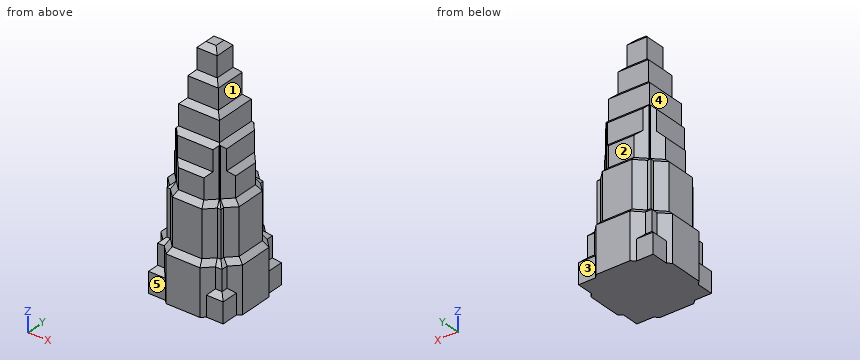
from build123d import *

# Parameters (mm, degrees)
F1_DEPTH     = 25.4
F2_SIZE      = 5.08
F3_DEPTH     = 25.4
F4_SIZE      = 5.08
F5_DEPTH     = 25.4
F6_DEPTH     = 25.4
F7_SIZE      = 5.08
F8_DEPTH     = 25.4
F9_SIZE      = 5.08
F10_DEPTH    = 25.4
F11_T1_DEPTH = 61.5024806542
F11_T3_DEPTH = 61.5024806542
F12_DEPTH    = 25.4
F13_SIZE     = 5.08
F14_DEPTH    = 25.4
F15_SIZE     = 5.08
F16_DEPTH    = 25.4
F17_SIZE     = 5.08


# Not quite as in the source:
# - a fillet or chamfer that OpenCascade refuses, or shapes differently, is made with other operations: its cross-section is extruded or revolved along the edge and cut away or added


with BuildPart() as f1:
    # F0 (on Top) → F1 (new body)
    with BuildSketch(Plane.XY):
        Polygon((37.0489656925, 20.3627443159), (37.0489656925, 37.0489656925), (20.3627443159, 37.0489656925), align=None)
        Polygon((40.5962094665, 16.8155005419), (37.0489656925, 20.3627443159), (37.0489656925, -20.3627443159), (40.5962094665, -16.8155005419), align=None)
        Polygon((37.0489656925, -20.3627443159), (37.0489656925, 20.3627443159), (20.3627443159, 37.0489656925), (-20.3627443159, 37.0489656925), (-37.0489656925, 20.3627443159), (-37.0489656925, -20.3627443159), (-20.3627443159, -37.0489656925), (20.3627443159, -37.0489656925), align=None)
        Polygon((-20.3627443159, 37.0489656925), (20.3627443159, 37.0489656925), (16.8155005419, 40.5962094665), (-16.8155005419, 40.5962094665), align=None)
        Polygon((37.0489656925, -37.0489656925), (37.0489656925, -20.3627443159), (20.3627443159, -37.0489656925), align=None)
        Polygon((-37.0489656925, 20.3627443159), (-20.3627443159, 37.0489656925), (-37.0489656925, 37.0489656925), align=None)
        Polygon((16.8155005419, -40.5962094665), (20.3627443159, -37.0489656925), (-20.3627443159, -37.0489656925), (-16.8155005419, -40.5962094665), align=None)
        Polygon((-37.0489656925, -20.3627443159), (-37.0489656925, 20.3627443159), (-40.5962094665, 16.8155005419), (-40.5962094665, -16.8155005419), align=None)
        Polygon((-37.0489656925, -37.0489656925), (-20.3627443159, -37.0489656925), (-37.0489656925, -20.3627443159), align=None)
    extrude(amount=F1_DEPTH)

    # F2
    f2_edges = [f1.edges().sort_by_distance(p)[0] for p in [
        (-28.705855, 37.048966, 25.4),
        (-37.048966, 28.705855, 25.4),
        (28.705855, 37.048966, 25.4),
        (37.048966, 28.705855, 25.4),
        (37.048966, -28.705855, 25.4),
        (28.705855, -37.048966, 25.4),
        (-28.705855, -37.048966, 25.4),
        (-37.048966, -28.705855, 25.4),
    ]]
    chamfer(f2_edges, length=F2_SIZE)

    # F3 (add): a face of the model
    f3_faces = [f1.faces().sort_by_distance(p)[0] for p in [
        (0, 0, 25.4),
    ]]
    extrude(f3_faces, amount=F3_DEPTH)

    # F4
    f4_edges = [f1.edges().sort_by_distance(p)[0] for p in [
        (-21.129122, 36.282588, 50.8),
        (-28.705855, 31.968966, 50.8),
        (-31.968966, 28.705855, 50.8),
        (-36.282588, 21.129122, 50.8),
        (-40.596209, 0, 50.8),
        (-36.282588, -21.129122, 50.8),
        (-31.968966, -28.705855, 50.8),
        (-28.705855, -31.968966, 50.8),
        (-21.129122, -36.282588, 50.8),
        (0, -40.596209, 50.8),
        (21.129122, -36.282588, 50.8),
        (28.705855, -31.968966, 50.8),
        (31.968966, -28.705855, 50.8),
        (36.282588, -21.129122, 50.8),
        (40.596209, 0, 50.8),
        (36.282588, 21.129122, 50.8),
        (31.968966, 28.705855, 50.8),
        (28.705855, 31.968966, 50.8),
        (21.129122, 36.282588, 50.8),
        (0, 40.596209, 50.8),
    ]]
    chamfer(f4_edges, length=F4_SIZE)

    # F5 (add): a face of the model
    f5_faces = [f1.faces().sort_by_distance(p)[0] for p in [
        (0, 0, 50.8),
    ]]
    extrude(f5_faces, amount=F5_DEPTH)

    # F6 (add): a face of the model
    f6_faces = [f1.faces().sort_by_distance(p)[0] for p in [
        (0, 0, 76.2),
    ]]
    extrude(f6_faces, amount=F6_DEPTH)

    # F7
    f7_edges = [f1.edges().sort_by_distance(p)[0] for p in [
        (-19.024918, 31.202588, 101.6),
        (-25.113753, 26.888966, 101.6),
        (0, 35.516209, 101.6),
        (-26.888966, 25.113753, 101.6),
        (19.024918, 31.202588, 101.6),
        (-31.202588, 19.024918, 101.6),
        (25.113753, 26.888966, 101.6),
        (-35.516209, 0, 101.6),
        (26.888966, 25.113753, 101.6),
        (-31.202588, -19.024918, 101.6),
        (31.202588, 19.024918, 101.6),
        (-26.888966, -25.113753, 101.6),
        (35.516209, 0, 101.6),
        (-25.113753, -26.888966, 101.6),
        (31.202588, -19.024918, 101.6),
        (-19.024918, -31.202588, 101.6),
        (26.888966, -25.113753, 101.6),
        (0, -35.516209, 101.6),
        (25.113753, -26.888966, 101.6),
        (19.024918, -31.202588, 101.6),
    ]]
    chamfer(f7_edges, length=F7_SIZE)

    # F8 (add): a face of the model
    f8_faces = [f1.faces().sort_by_distance(p)[0] for p in [
        (0, 0, 101.6),
    ]]
    extrude(f8_faces, amount=F8_DEPTH)

    # F9
    f9_edges = [f1.edges().sort_by_distance(p)[0] for p in [
        (0, 30.436209, 127),
        (-30.436209, 0, 127),
        (30.436209, 0, 127),
        (0, -30.436209, 127),
    ]]
    chamfer(f9_edges, length=F9_SIZE)

    # F10 (add): a face of the model
    f10_faces = [f1.faces().sort_by_distance(p)[0] for p in [
        (0, 0, 127),
    ]]
    extrude(f10_faces, amount=F10_DEPTH)

    # F11: chamfer of 5.08 on 4 edges, made by hand

    # F11_s2 → F11_t1 (cut)
    with BuildSketch(Plane.XZ.offset(-30.7512403271)):
        Polygon((-25.3562094665, 147.32), (-20.2762094665, 152.4), (-25.3562094665, 152.4), align=None)
        Polygon((25.3562094665, 147.32), (20.2762094665, 152.4), (25.3562094665, 152.4), align=None)
    extrude(amount=F11_T1_DEPTH, mode=Mode.SUBTRACT)

    # F11_s4 → F11_t3 (cut)
    with BuildSketch(Plane.YZ.offset(-30.7512403271)):
        Polygon((-25.3562094665, 147.32), (-20.2762094665, 152.4), (-25.3562094665, 152.4), align=None)
        Polygon((20.2762094665, 152.4), (25.3562094665, 147.32), (25.3562094665, 152.4), align=None)
    extrude(amount=F11_T3_DEPTH, mode=Mode.SUBTRACT)

    # F12 (add): a face of the model
    f12_faces = [f1.faces().sort_by_distance(p)[0] for p in [
        (0, 0, 152.4),
    ]]
    extrude(f12_faces, amount=F12_DEPTH)

    # F13
    f13_edges = [f1.edges().sort_by_distance(p)[0] for p in [
        (0, 20.276209, 177.8),
        (20.276209, 0, 177.8),
        (0, -20.276209, 177.8),
        (-20.276209, 0, 177.8),
    ]]
    chamfer(f13_edges, length=F13_SIZE)

    # F14 (add): a face of the model
    f14_faces = [f1.faces().sort_by_distance(p)[0] for p in [
        (0, 0, 177.8),
    ]]
    extrude(f14_faces, amount=F14_DEPTH)

    # F15
    f15_edges = [f1.edges().sort_by_distance(p)[0] for p in [
        (0, 15.196209, 203.2),
        (-15.196209, 0, 203.2),
        (15.196209, 0, 203.2),
        (0, -15.196209, 203.2),
    ]]
    chamfer(f15_edges, length=F15_SIZE)

    # F16 (add): a face of the model
    f16_faces = [f1.faces().sort_by_distance(p)[0] for p in [
        (0, 0, 203.2),
    ]]
    extrude(f16_faces, amount=F16_DEPTH)

    # F17
    f17_edges = [f1.edges().sort_by_distance(p)[0] for p in [
        (0, 10.116209, 228.6),
        (-10.116209, 0, 228.6),
        (10.116209, 0, 228.6),
        (0, -10.116209, 228.6),
    ]]
    chamfer(f17_edges, length=F17_SIZE)


solid = f1.part
CAD build for the part. Positions are in the model's coordinates, mm. Face numbers are marked on the shaded views. A direction names the side the tool comes from. Give positions to 0.01 mm unless a question says otherwise; leave off trailing zeros. Order: outer loops, then holes, each group sorted by start corner. A loop starts at its lowest first (then second) coordinate and runs counter-clockwise, first axis right, second up. Notation, with made-up numbers: (37.5, -3.75) - (63.5, -3.75) arc R21 ccw to (63.5, 4.25) - close; hole circle Ø6 at (83.5, 78.25). An arc over 180 degrees is marked (long way). Answer in a Markdown table with one row per item.
1. Saw through at B-B, the plane z = 74. Give the cut face in (x, y), plus the area to 3 significant figures.
Data:
| item | result |
|---|---|
| outline | (-35.52, -14.71) - (-26.89, -23.34) - (-26.89, -26.89) - (-23.34, -26.89) - (-14.71, -35.52) - (14.71, -35.52) - (23.34, -26.89) - (26.89, -26.89) - (26.89, -23.34) - (35.52, -14.71) - (35.52, 14.71) - (26.89, 23.34) - (26.89, 26.89) - (23.34, 26.89) - (14.71, 35.52) - (-14.71, 35.52) - (-23.34, 26.89) - (-26.89, 26.89) - (-26.89, 23.34) - (-35.52, 14.71) - close |
| area | 4,210 mm² |
2. Saw through at C-C, the plane z = 212. Give the cut face in (x, y), plus the area to 3 significant figures.
Data:
| item | result |
|---|---|
| outline | (-10.12, -10.12) - (10.12, -10.12) - (10.12, 10.12) - (-10.12, 10.12) - close |
| area | 409 mm² |
3. Tool access for the marked faces 1, 2, 3, 4 and 5: list every direction of +Z, -Z, +X, -X, +Y, -Y with a clear straight run to the whole face (end or side of a thin tool).
Data:
| item | result |
|---|---|
| face 1 | +Z, +X, +Y, -Y |
| face 2 | +Z, +X, -X, +Y |
| face 3 | +Z, -Z, +X, +Y |
| face 4 | +Z, -X, +Y, -Y |
| face 5 | +Z, -Z, -X, -Y |
4. Flat gauge pins, fed straight in: pin 1 (22.5 mm diameter, centred on y = 4.5, z = 189.5, fed in from +X); pin 2 (22.5 mm diameter, centred on y = 3.5, z = 213, fed in from -X); pin 3 (3 mm diameter, centred on x = -5.5, y = -20.5, fed in from +Z). Where does each tip first touch, or does it go through?
Data:
| item | result |
|---|---|
| pin 1 | stops at x = 15.2 |
| pin 2 | stops at x = -11.57 |
| pin 3 | stops at z = 174 |
5. Saw through at D-D, the plane z = 124.5. Give the cut face in (x, y).
Data:
| item | result |
|---|---|
| outline | (-27.86, -15.19) - (-21.81, -21.23) - (-21.81, -21.81) - (-21.23, -21.81) - (-15.19, -27.86) - (15.19, -27.86) - (21.23, -21.81) - (21.81, -21.81) - (21.81, -21.23) - (27.86, -15.19) - (27.86, 15.19) - (21.81, 21.23) - (21.81, 21.81) - (21.23, 21.81) - (15.19, 27.86) - (-15.19, 27.86) - (-21.23, 21.81) - (-21.81, 21.81) - (-21.81, 21.23) - (-27.86, 15.19) - close |
6. Probe probe 1 along Y at (x, z) = (-8, 172); probe 2 along Y at (x, z) = (-32.5, 70). List the from-to ranges inside material, lowest first. Write a range as [from, to].
Data:
| item | result |
|---|---|
| probe 1 | y = [-20.28, 20.28] |
| probe 2 | y = [-17.73, 17.73] |
